from build123d import *

# Parameters (mm, degrees)
BOSS_EXTRUDE1_DEPTH = 1.45
SKETCH2_R           = 4
BOSS_EXTRUDE2_DEPTH = 3
SKETCH3_R           = 1.625
CUT_EXTRUDE1_DEPTH  = 20.460360465


with BuildPart() as part:
    # Sketch1 → Boss-Extrude1 (new, symmetric)
    with BuildSketch(Plane(origin=(0, 0, 0), x_dir=(1, 0, 0), z_dir=(0, 1, 0))):
        with BuildLine():
            Line((-14.075, 4), (14.075, 4))
            ThreePointArc((14.075, 4), (18.075, 0), (14.075, -4))
            Line((14.075, -4), (-14.075, -4))
            ThreePointArc((-14.075, -4), (-18.075, 0), (-14.075, 4))
        make_face()
    extrude(amount=BOSS_EXTRUDE1_DEPTH, both=True)

    # Sketch2 → Boss-Extrude2 (add, symmetric)
    with BuildSketch(Plane(origin=(0, 0, 0), x_dir=(1, 0, 0), z_dir=(0, 1, 0))):
        with Locations(Location((-14.075, 0, 0), (0, 0, 270))):
            Circle(SKETCH2_R)
        with Locations(Location((14.075, 0, 0), (0, 0, 270))):
            Circle(SKETCH2_R)
    extrude(amount=BOSS_EXTRUDE2_DEPTH, both=True)

    # Fillet1: read off the stored shape, not the designer's step
    # Fillet1 outline → Fillet1 (revolve, cut)
    with BuildSketch(Plane(origin=(14.075, 0, 0), x_dir=(1, 0, 0), z_dir=(0, 0, 1))):
        with BuildLine():
            ThreePointArc((3, 3), (3.707106781, 2.707106781), (4, 2))
            Line((4, 2), (4, 3))
            Line((4, 3), (3, 3))
        make_face()
        with BuildLine():
            Line((4, -3), (4, -2))
            ThreePointArc((4, -2), (3.707106781, -2.707106781), (3, -3))
            Line((3, -3), (4, -3))
        make_face()
    revolve(axis=Axis((14.075, 0, 0), (0, 1, 0)), mode=Mode.SUBTRACT)

    # Fillet1 2 outline → Fillet1 2 (revolve, cut)
    with BuildSketch(Plane(origin=(-14.075, 0, 0), x_dir=(1, 0, 0), z_dir=(0, 0, 1))):
        with BuildLine():
            ThreePointArc((4, -2), (3.707106781, -2.707106781), (3, -3))
            Line((3, -3), (4, -3))
            Line((4, -3), (4, -2))
        make_face()
        with BuildLine():
            ThreePointArc((3, 3), (3.707106781, 2.707106781), (4, 2))
            Line((4, 2), (4, 3))
            Line((4, 3), (3, 3))
        make_face()
    revolve(axis=Axis((-14.075, 0, 0), (0, 1, 0)), mode=Mode.SUBTRACT)

    # Sketch3 → Cut-Extrude1 (cut, through all)
    with BuildSketch(Plane(origin=(0, 3, 0), x_dir=(1, 0, 0), z_dir=(0, 1, 0))):
        with Locations(Location((-14.075, 0, 0), (0, 0, 270))):
            Circle(SKETCH3_R)
        with Locations(Location((14.075, 0, 0), (0, 0, 270))):
            Circle(SKETCH3_R)
    extrude(amount=-CUT_EXTRUDE1_DEPTH, mode=Mode.SUBTRACT)


solid = part.part
Input: part model. Units: mm. Frame: model coordinates. Coordinates: 2 decimals unless noted, no trailing zeros. Order: outer loops, then holes, each group sorted by start corner. A loop starts at its lowest first (then second) coordinate and runs counter-clockwise, first axis right, second up. Notation, with made-up numbers: M -25.5,50.25 L 18.5,50.25 A11 cw 18.5,61.25 Z; hole C 47,37.5 d3. An arc over 180 degrees is marked long. Write item = value, one per line. Start each with the question number.
(1) Line query: line 1 along X through (y, z) = (-1.25, 0) (3 decimals); line 2 along X through (y, z) = (1.6, 0) (3 decimals); line 3 along X through (y, z) = (-1.5, -1). Output: solid intervals per line, ascending. Write a range as [from, to].
(2) Section A-A on z = 0. Output: boundary loops of the cut face in (x, y) (3 decimals).
(3) Section B-B on y = 0.5. Output: boundary loops of the cut face in (x, z) (3 decimals).
(4) Section C-C on x = 5. Output: boundary loops of the cut face in (y, z), and give its area (3 significant figures).
(5) Pull-direction query (X, two-part tool) for faces 1 (the cylindrical face through (15.686, 0.042, -0.212)), 2 (the flat face through (-15.4, 3, 1.3)), 3 (the flat face through (0, -1.45, 0)); classes: released by +X, released by -X, zero draft, split by the parting line, or undercut.
(6) First-contact query: P1, Ø1.9, axis at x = -14.075, z = 0, coming from the +Y side; P2, Ø4, axis at x = -3.5, z = -1.5, coming from the -Y side; P3, Ø1, axis at y = 0, z = 3, coming from the -X side; P4, Ø1, axis at x = -2, z = 3, coming from the +Y side. Flat tips, straight axial feed; report the tip coordinate or a pass-through.
Result set:
q1.line_1 = [-18.075, -15.7], [-12.45, 12.45], [15.7, 18.075]
q1.line_2 = [-18.075, -15.7], [-12.45, -10.075], [10.075, 12.45], [15.7, 18.075]
q1.line_3 = [-17.95, -15.36], [-12.79, -10.2], [10.2, 12.79], [15.36, 17.95]
q2.outline = M -18.075,-2 A1 ccw -17.075,-3 L -15.7,-3 L -15.7,3 L -17.075,3 A1 ccw -18.075,2 Z; M -12.45,-3 L -11.075,-3 A1 ccw -10.075,-2 L -10.075,-1.45 L 10.075,-1.45 L 10.075,-2 A1 ccw 11.075,-3 L 12.45,-3 L 12.45,3 L 11.075,3 A1 ccw 10.075,2 L 10.075,1.45 L -10.075,1.45 L -10.075,2 A1 ccw -11.075,3 L -12.45,3 Z; M 15.7,-3 L 17.075,-3 A1 ccw 18.075,-2 L 18.075,2 A1 ccw 17.075,3 L 15.7,3 Z
q3.outline = M -14.075,-4 L 14.075,-4 A4 ccw 14.075,4 L -14.075,4 A4 ccw Z; hole C -14.075,0 d3.25; hole C 14.075,0 d3.25
q4.outline = M -1.45,-4 L 1.45,-4 L 1.45,4 L -1.45,4 Z
q4.area = 23.2 mm²
q5.face_1 = undercut
q5.face_2 = zero draft
q5.face_3 = undercut
q6.P1 = through
q6.P2 = -1.45
q6.P3 = -17.2
q6.P4 = 1.45
